Build history of the part. All positions in model axes, mm. Face numbers are marked on the shaded views. A direction names the side the tool comes from. Coordinates: 2 decimals unless noted, no trailing zeros. Order: outer loops, then holes, each group sorted by start corner. A loop starts at its lowest first (then second) coordinate and runs counter-clockwise, first axis right, second up. Notation, with made-up numbers: (-22.75, 1) - (4.25, 1) arc R28 ccw to (4.25, 22) - close; hole circle Ø11 at (-34, 71). An arc over 180 degrees is marked (long way). Write each question's results on one line, items separated by ' | '. Start each with the question number.
from build123d import *

# Parameters (mm, degrees)
SKETCH2_R           = 11
SKETCH2_R_2         = 1.15
BOSS_EXTRUDE1_DEPTH = 20
CHAMFER1_SIZE       = 3
SKETCH5_R           = 2
CUT_EXTRUDE2_DEPTH  = 14.5
SKETCH6_R           = 2
CUT_EXTRUDE3_DEPTH  = 8
CHAMFER2_SIZE       = 0.3
CHAMFER2_SIZE2      = 1.2
SKETCH7_W           = 1
SKETCH7_H           = 3
CUT_EXTRUDE4_DEPTH  = 1


with BuildPart() as part:
    # Sketch2 → Boss-Extrude1 (new body)
    with BuildSketch(Plane(origin=(0, 0, 0), x_dir=(0, 0, -1), z_dir=(1, 0, 0))):
        Circle(SKETCH2_R)
        with Locations((0, 6)):
            Circle(SKETCH2_R_2, mode=Mode.SUBTRACT)
        with Locations((-6, 0)):
            Circle(SKETCH2_R_2, mode=Mode.SUBTRACT)
        with Locations((0, -6)):
            Circle(SKETCH2_R_2, mode=Mode.SUBTRACT)
        with Locations((6, 0)):
            Circle(SKETCH2_R_2, mode=Mode.SUBTRACT)
    extrude(amount=BOSS_EXTRUDE1_DEPTH)

    # Chamfer1
    chamfer1_edges = [part.edges().sort_by_distance(p)[0] for p in [
        (20, 0, 11),
    ]]
    chamfer(chamfer1_edges, length=CHAMFER1_SIZE)

    # Sketch5 → Cut-Extrude2 (cut)
    with BuildSketch(Plane.ZY):
        with Locations((-6, 0)):
            Circle(SKETCH5_R)
        with Locations((0, 6)):
            Circle(SKETCH5_R)
        with Locations((0, -6)):
            Circle(SKETCH5_R)
        with Locations((6, 0)):
            Circle(SKETCH5_R)
    extrude(amount=-CUT_EXTRUDE2_DEPTH, mode=Mode.SUBTRACT)

    # Sketch6 → Cut-Extrude3 (cut)
    with BuildSketch(Plane.ZY):
        with Locations((5.303300859, 5.303300859)):
            Circle(SKETCH6_R)
        with Locations((-5.303300859, 5.303300859)):
            Circle(SKETCH6_R)
        with Locations((-5.303300859, -5.303300859)):
            Circle(SKETCH6_R)
        with Locations((5.303300859, -5.303300859)):
            Circle(SKETCH6_R)
    extrude(amount=-CUT_EXTRUDE3_DEPTH, mode=Mode.SUBTRACT)

    # Chamfer2
    chamfer2_edges = [part.edges().sort_by_distance(p)[0] for p in [
        (0, -5.303300859, 3.303300859),
        (0, -5.303300859, -7.303300859),
        (0, 5.303300859, -7.303300859),
        (0, 5.303300859, 3.303300859),
    ]]
    chamfer2_side = [part.faces().sort_by_distance(p)[0] for p in [
        (0, 0, 0),
    ]]
    chamfer(chamfer2_edges, length=CHAMFER2_SIZE, length2=CHAMFER2_SIZE2, reference=chamfer2_side[0])

    # Sketch7 → Cut-Extrude4 (cut)
    with BuildSketch(Plane.ZY):
        with Locations((0, 11)):
            Rectangle(SKETCH7_W, SKETCH7_H)
    extrude(amount=-CUT_EXTRUDE4_DEPTH, mode=Mode.SUBTRACT)


solid = part.part
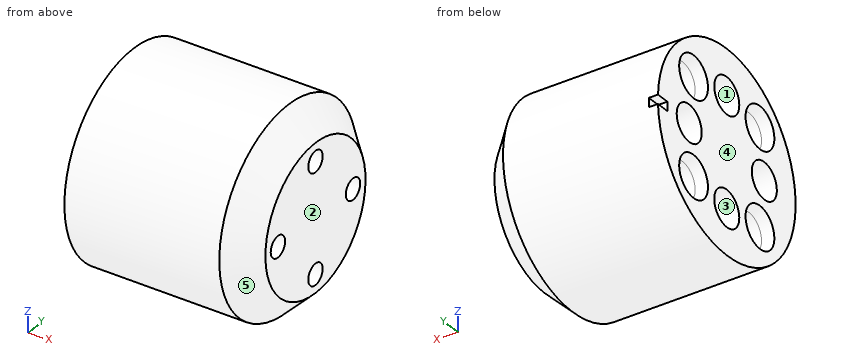
Item 1: Slice it at B-B (z = 0). Write the cut outline in (x, y), then the cut area to 3 significant figures.
Item 2: Probe probe 1 along Y at (x, z) = (6.25, 6.25); probe 2 along Y at (x, z) = (7.5, 4.75). List the from-to ranges inside material, lowest first.
Item 3: Slice it at C-C (x = 2.75). Count the separate pieces of the cut face and the enclosed holes in it, then the cut area to 3 significant figures.
Item 4: Pull direction Y, two halves, no side cores. Call the marked faces 3, 4 and 5: released by +Y, released by -Y, zero draft, split by the parting line, or undercut.
Item 5: Flat gauge pins, fed straight in: P1, Ø3, axis at y = -6, z = 0, coming from the -X side; P2, Ø1, axis at x = 6, y = -4.5, coming from the +Z side; P3, Ø2.5, axis at y = -5.3, z = 5.3, coming from the -X side. Where does each tip first touch, or does it go through?
Item 6: Slice it at A-A (y = 0). Write the cut outline in (x, z).
Item 7: Which spindle directions (+Z, -Z, +X, -X, +Y, -Y) get a long thin tool onto all of the face, cutting with end or side? Do the marked faces 1 and 2. Say none if no direction does.
Item 8: Slice it at D-D (x = 18.75). Write the cut outline in (y, z), then the cut area to 3 significant figures.
Resolved:
1) outline: (0, -11) - (17, -11) - (20, -8) - (20, -7.15) - (14.5, -7.15) - (14.5, -8) - (0, -8) - close; (0, -4) - (14.5, -4) - (14.5, -4.85) - (20, -4.85) - (20, 4.85) - (14.5, 4.85) - (14.5, 4) - (0, 4) - close; (0, 8) - (14.5, 8) - (14.5, 7.15) - (20, 7.15) - (20, 8) - (17, 11) - (1, 11) - (1, 9.5) - (0, 9.5) - close | area: 288 mm^2
2) probe 1: -9.05 to -7.07, -3.54 to -1.98, 1.98 to 3.54, 7.07 to 9.05 | probe 2: -9.92 to -7.23, -3.38 to -1.56, 1.56 to 3.38, 7.23 to 9.92
3) separate pieces: 1 | enclosed holes: 8 | area: 280 mm^2
4) face 3: undercut | face 4: zero draft | face 5: split by the parting line
5) P1: x = 14.5 | P2: z = 10.25 | P3: x = 8
6) outline: (0, -11) - (17, -11) - (20, -8) - (20, -7.15) - (14.5, -7.15) - (14.5, -8) - (0, -8) - close; (0, -4) - (14.5, -4) - (14.5, -4.85) - (20, -4.85) - (20, 4.85) - (14.5, 4.85) - (14.5, 4) - (0, 4) - close; (0, 8) - (14.5, 8) - (14.5, 7.15) - (20, 7.15) - (20, 8) - (17, 11) - (0, 11) - close
7) face 1: -X | face 2: +Z, -Z, +X, +Y, -Y
8) outline: circle Ø18.5 at (0, 0); hole circle Ø2.3 at (-6, 0); hole circle Ø2.3 at (0, -6); hole circle Ø2.3 at (0, 6); hole circle Ø2.3 at (6, 0) | area: 252 mm^2
